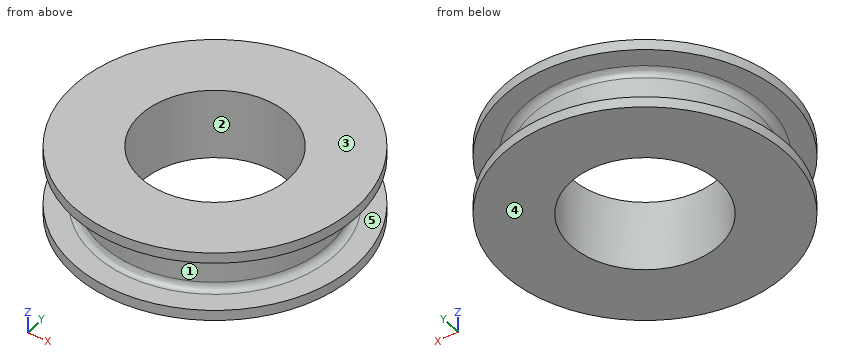
```python
from build123d import *

# Parameters (mm, degrees)
SKETCH_1_R      = 40
SKETCH_1_R_2    = 30
SKETCH_1_R_3    = 21
EXTRUDE_1_DEPTH = 10


with BuildPart() as part:
    # 草图1 → 凸台-拉伸1 (new, symmetric)
    with BuildSketch(Plane.XY):
        Circle(SKETCH_1_R)
        Circle(SKETCH_1_R_2, mode=Mode.SUBTRACT)
        Circle(SKETCH_1_R_2)
        Circle(SKETCH_1_R_3, mode=Mode.SUBTRACT)
    extrude(amount=EXTRUDE_1_DEPTH, both=True)

    # 草图2 → 切除-旋转1 (revolve, cut)
    with BuildSketch(Plane(origin=(0, 0, 0), x_dir=(0, 0, -1), z_dir=(1, 0, 0)), mode=Mode.PRIVATE) as cut_revolve_1_sk:
        with BuildLine():
            Line((-7, 40), (-7, 34))
            ThreePointArc((-7, 34), (-6.414213562, 32.585786438), (-5, 32))
            Line((-5, 32), (5, 32))
            ThreePointArc((5, 32), (6.414213562, 32.585786438), (7, 34))
            Line((7, 34), (7, 40))
            Line((7, 40), (-7, 40))
        make_face()
    revolve(cut_revolve_1_sk.sketch.rotate(Axis((0, 0, 0), (0, 0, 1)), 90), axis=Axis((0, 0, 0), (0, 0, 1)), mode=Mode.SUBTRACT)


solid = part.part
```
Read the model definition and answer for the solid it produces. Units are mm, in the model's axes. Face numbers are marked on the shaded views. A direction names the side the tool comes from. Coordinates: 2 decimals unless noted, no trailing zeros. Loops run counter-clockwise (first coordinate to the right, second up) from the corner with the lowest first, then second, coordinate; pieces in that order, holes last. Notation, with made-up numbers: (88, 54.25) - (124, 54.25) arc R13 cw to (124, 58.25) - close; hole circle Ø4 at (81.25, 86.25). An arc over 180 degrees is marked (long way). Answer in a Markdown table with one row per item.
1. Find section C-C, the plane z = 1.75. Write down the section's boundary in (x, y).
Conclusion:
| item | result |
|---|---|
| outline | circle Ø64 at (0, 0); hole circle Ø42 at (0, 0) |
2. Determine the mould class of the marked faces 3, 4 and 5 for opening direction Z: +Z half, -Z half, draft (parallel to the pull), parting line (faces both ways), or undercut.
Conclusion:
| item | result |
|---|---|
| face 3 | +Z half |
| face 4 | -Z half |
| face 5 | undercut |
3. Given pin 1 (12 mm diameter, centred on y = -10.5, z = 2.5, fed in from +X); pin 2 (3 mm diameter, centred on x = 10, z = -7.5, fed in from +Y); pin 3 (25 mm diameter, centred on x = 0, y = 0, fed in from -Z); pin 4 (1.5 mm diameter, centred on y = 7.5, z = -7, fed in from -X), each flat-ended and moving along its own axis, determine where each tip first touches the part or whether it passes through.
Conclusion:
| item | result |
|---|---|
| pin 1 | stops at x = 39.46 |
| pin 2 | stops at y = 39.09 |
| pin 3 | passes through |
| pin 4 | stops at x = -39.43 |
4. Straight lines are drawn through the part: line 1 (Y direction, x = 0, z = 3.25); line 2 (Z direction, x = 20, y = -28.5); line 3 (X direction, y = 6, z = 6.25). For each, find the intervals that lie inside material, in ascending order.
Conclusion:
| item | result |
|---|---|
| line 1 | y = -32 to -21, 21 to 32 |
| line 2 | z = -10 to -7, 7 to 10 |
| line 3 | x = -31.88 to -20.12, 20.12 to 31.88 |
5. Which of the six approach directions +Z, -Z, +X, -X, +Y, -Y give full straight-line access (tool end or side, diameter ignored) to the marked faces 1 and 2?
Conclusion:
| item | result |
|---|---|
| face 1 | none |
| face 2 | +Z, -Z |
6. Find section A-A, the plane y = 0. Write down the section's boundary in (x, z).
Conclusion:
| item | result |
|---|---|
| outline | (-40, -10) - (-21, -10) - (-21, 10) - (-40, 10) - (-40, 7) - (-34, 7) arc R2 cw to (-32, 5) - (-32, -5) arc R2 cw to (-34, -7) - (-40, -7) - close; (21, -10) - (40, -10) - (40, -7) - (34, -7) arc R2 cw to (32, -5) - (32, 5) arc R2 cw to (34, 7) - (40, 7) - (40, 10) - (21, 10) - close |
